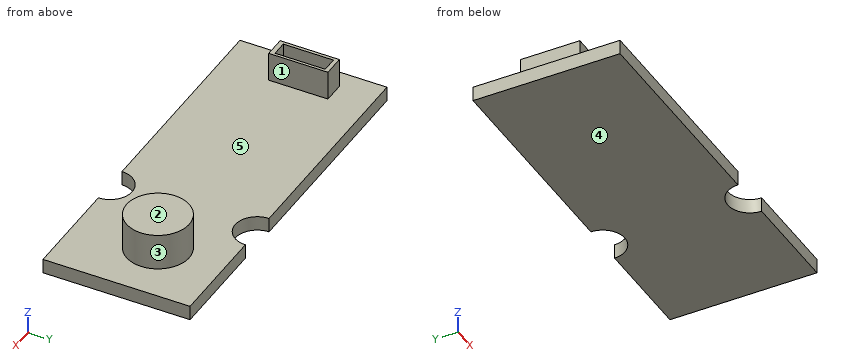
```python
from build123d import *

# Parameters (mm, degrees)
ESQUISSE1_W             = 50
ESQUISSE1_H             = 20
BOSS_EXTRU_1_DEPTH      = 2
ESQUISSE2_R             = 4.260694663
BOSS_EXTRU_2_DEPTH      = 5
ESQUISSE3_R             = 3
ENL_V_MAT_EXTRU_1_DEPTH = 8
ESQUISSE4_W             = 2.90032215
ESQUISSE4_H             = 8.050990352
BOSS_EXTRU_3_DEPTH      = 4
ESQUISSE5_W             = 2.093863404
ESQUISSE5_H             = 6.825994699
ENL_V_MAT_EXTRU_2_DEPTH = 3


with BuildPart() as part:
    # Esquisse1 → Boss.-Extru.1 (new body)
    with BuildSketch(Plane.XY):
        with Locations((3.888470464, 6.071428571)):
            Rectangle(ESQUISSE1_W, ESQUISSE1_H)
    extrude(amount=BOSS_EXTRU_1_DEPTH)

    # Esquisse2 → Boss.-Extru.2 (add)
    with BuildSketch(Plane.XY.offset(2)):
        with Locations((20.32390926, 7.113111312)):
            Circle(ESQUISSE2_R)
    extrude(amount=BOSS_EXTRU_2_DEPTH)

    # Esquisse3 → Enlèv. mat.-Extru.1 (cut)
    with BuildSketch(Plane.XY.offset(2)):
        with Locations((11.836123966, 16.071428571)):
            Circle(ESQUISSE3_R)
        with Locations((11.836123966, -3.928571429)):
            Circle(ESQUISSE3_R)
    extrude(amount=-ENL_V_MAT_EXTRU_1_DEPTH, mode=Mode.SUBTRACT)

    # Esquisse4 → Boss.-Extru.3 (add)
    with BuildSketch(Plane.XY.offset(2)):
        with Locations((-17.118363615, 6.928845047)):
            Rectangle(ESQUISSE4_W, ESQUISSE4_H)
    extrude(amount=BOSS_EXTRU_3_DEPTH)

    # Esquisse5 → Enlèv. mat.-Extru.2 (cut)
    with BuildSketch(Plane.XY.offset(6)):
        with Locations((-17.095752138, 6.967080934)):
            Rectangle(ESQUISSE5_W, ESQUISSE5_H)
    extrude(amount=-ENL_V_MAT_EXTRU_2_DEPTH, mode=Mode.SUBTRACT)


solid = part.part
```
Model file for the job. Use its own axes, mm. Face numbers are marked on the shaded views. A direction names the side the tool comes from. Coordinates: 2 decimals unless noted, no trailing zeros. Write each loop counter-clockwise with the first axis right and the second up, starting at its lowest first coordinate (ties: lowest second). Pieces come first, ordered by that corner, then holes. Notation, with made-up numbers: (76.5, 66) - (106.5, 66) arc R24 ccw to (106.5, 98) - close; hole circle Ø11 at (74, 65.5). An arc over 180 degrees is marked (long way). One line per item, written item: value. Start each with the question number.
1. Slice it at B-B (y = -2.25). Write the cut outline in (x, z), plus the area to 3 significant figures.
2. Probe line 1 (X direction, y = 5.75, z = 5.5); line 2 (Z direction, x = 9, y = 8.75); line 3 (X direction, y = -1.5, z = 1). List the from-to ranges inside material, lowest first. Write a range as from..to.
3. Flat gauge pins, fed straight in: pin 1 (4 mm diameter, centred on x = -11.5, z = 4.5, fed in from -Y); pin 2 (1.5 mm diameter, centred on y = 6.5, z = 4, fed in from +X); pin 3 (1.2 mm diameter, centred on y = 8, z = 3, fed in from -X); pin 4 (1.7 mm diameter, centred on x = -17, z = 4, fed in from -Y). Where does each tip first touch, or does it go through?
4. Tool access for the marked faces 1, 2 and 3: list every direction of +Z, -Z, +X, -X, +Y, -Y with a clear straight run to the whole face (end or side of a thin tool).
5. Slice it at C-C (z = 4). Write the cut outline in (x, y).
6. Slice it at A-A (z = 1.25). Write the cut outline in (x, y).
7. Slice it at D-D (x = 20). Write the cut outline in (y, z).
8. Mould opens along X. For the marked faces 4 and 5 say: released by +X, released by -X, zero draft, split by the parting line, or undercut.
Answers below:
1. outline: (-21.11, 0) - (9.35, 0) - (9.35, 2) - (-21.11, 2) - close; (14.32, 0) - (28.89, 0) - (28.89, 2) - (14.32, 2) - close
1. area: 90.1 mm^2
2. line 1: x = -18.57..-18.14, -16.05..-15.67, 16.29..24.36
2. line 2: z = 0..2
2. line 3: x = -21.11..10.07, 13.6..28.89
3. pin 1: passes through
3. pin 2: stops at x = 24.58
3. pin 3: stops at x = -18.57
3. pin 4: stops at y = 2.9
4. face 1: +Z, +Y, -Y
4. face 2: +Z, +X, -X, +Y, -Y
4. face 3: +Z
5. outline: (-18.57, 2.9) - (-15.67, 2.9) - (-15.67, 10.95) - (-18.57, 10.95) - close; circle Ø8.52 at (20.32, 7.11); hole (-18.14, 3.55) - (-16.05, 3.55) - (-16.05, 10.38) - (-18.14, 10.38) - close
6. outline: (-21.11, -3.93) - (8.84, -3.93) arc R3 cw to (14.84, -3.93) - (28.89, -3.93) - (28.89, 16.07) - (14.84, 16.07) arc R3 cw to (8.84, 16.07) - (-21.11, 16.07) - close
7. outline: (-3.93, 0) - (16.07, 0) - (16.07, 2) - (11.36, 2) - (11.36, 7) - (2.86, 7) - (2.86, 2) - (-3.93, 2) - close
8. face 4: zero draft
8. face 5: undercut
